Check sheet for the drawn part. Datum: minimum x, y, z corner. Units: mm. A direction names the side the tool comes from. Round coordinates to 2 decimals unless told otherwise and drop trailing zeros. Write each loop counter-clockwise with the first axis right and the second up, starting at its lowest first coordinate (ties: lowest second). Pieces come first, ordered by that corner, then holes. Notation, with made-up numbers: M 34,37.5 L 45,37.5 A20 cw 45,44.5 Z; hole C -19,88 d3. An arc over 180 degrees is marked long. Answer in a Markdown table with one row per item. Add a question column.
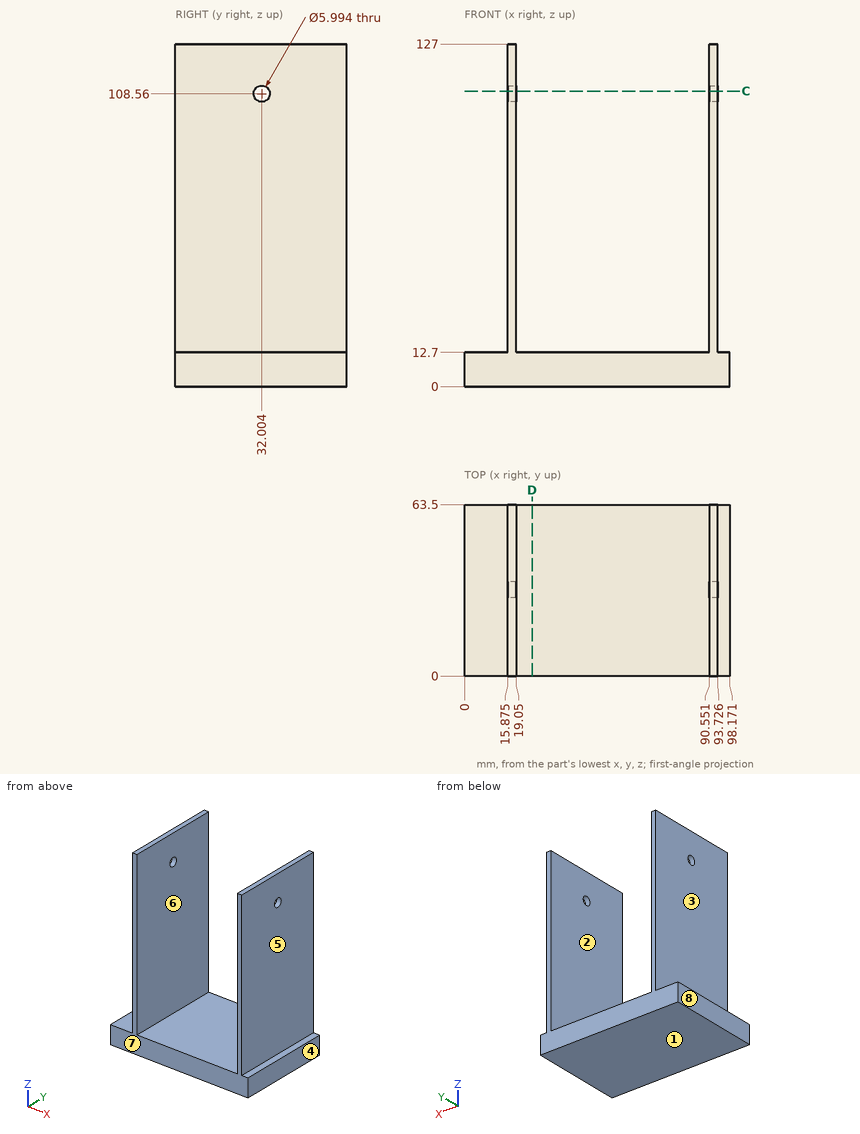
Item 1: Mould release check, pull along X, two halves, no side actions. Record for the marked faces 6, 7 and 8: +X half, -X half, draft (parallel to the pull), parting line (faces both ways), or undercut.
Item 2: Section check C-C, the plane z = 109.5. Give the number of separate pieces and of enclosed holes in the cut face, and give its area (3 significant figures).
Item 3: Scan lines: probe 1 along Z at (x, y) = (56.5, 51); probe 2 along Y at (x, z) = (18, 106.5) (1 decimal). Record each from-to range of solid material in increasing order. Write a range as from..to.
Item 4: Gauge pin test, flat ends, axial feed: pin 1 Ø19 at (y, z) = (40, 61) entering from -X (3 decimals); pin 2 Ø19 at (y, z) = (31, 89.5) entering from +X; pin 3 Ø12.5 at (x, y) = (7, 46.5) entering from +Z. Record the tip position at first contact, or that the pin passes through.
Item 5: Section check D-D, the plane x = 25. Record the boundary of the cut face in (y, z).
Item 6: Access from +Z, -Z, +X, -X, +Y, -Y to the whole of each face (thin tool, end or side, straight path). Record for the marked faces 1, 2, 3, 4 and 5.
Result sheet:
| question | item | result |
|---|---|---|
| 1 | face 6 | undercut |
| 1 | face 7 | draft |
| 1 | face 8 | -X half |
| 2 | separate pieces | 4 |
| 2 | enclosed holes | 0 |
| 2 | area | 367 mm^2 |
| 3 | probe 1 | z = 0..12.7 |
| 3 | probe 2 | y = 0..29.8, 34.2..63.5 |
| 4 | pin 1 | stops at x = 15.875 |
| 4 | pin 2 | stops at x = 93.73 |
| 4 | pin 3 | stops at z = 12.7 |
| 5 | outline | M 0,0 L 63.5,0 L 63.5,12.7 L 0,12.7 Z |
| 6 | face 1 | -Z, +X, -X, +Y, -Y |
| 6 | face 2 | +Z, +Y, -Y |
| 6 | face 3 | +Z, -X, +Y, -Y |
| 6 | face 4 | +Z, -Z, +X, +Y, -Y |
| 6 | face 5 | +Z, +X, +Y, -Y |
